```python
from build123d import *

# Parameters (mm, degrees)
F1_DEPTH = 0.5
F4_SCALE = 3


with BuildPart() as f1:
    # F0 (on Top) → F1 (new body)
    with BuildSketch(Plane.XY):
        with BuildLine():
            ThreePointArc((0.6081234737, 2.1142814502), (-0.4630317257, 1.4250651194), (-1.7347256805, 1.3530436147))
            ThreePointArc((-1.7347256805, 1.3530436147), (-1.7798374262, 1.2931275831), (-1.8228806624, 1.2317086913))
            ThreePointArc((-1.8228806624, 1.2317086913), (-1.4984021401, 0), (-1.8228806624, -1.2317086913))
            ThreePointArc((-1.8228806624, -1.2317086913), (-1.7798374262, -1.2931275831), (-1.7347256805, -1.3530436147))
            ThreePointArc((-1.7347256805, -1.3530436147), (-0.4646832841, -1.4263763437), (0.6048373994, -2.1152238487))
            ThreePointArc((0.6048373994, -2.1152238487), (0.6802746399, -2.0921822636), (0.7548374053, -2.0664512337))
            ThreePointArc((0.7548374053, -2.0664512337), (1.2149085882, -0.8808585803), (2.1987212669, -0.075000003))
            ThreePointArc((2.1987212669, -0.075000003), (2.2000000477, 0), (2.1987212669, 0.075000003))
            ThreePointArc((2.1987212669, 0.075000003), (1.2122351514, 0.8807449808), (0.7507612307, 2.0679356335))
            ThreePointArc((0.7507612307, 2.0679356335), (0.6798374024, 2.0923243812), (0.6081234737, 2.1142814502))
        make_face()
        with BuildLine():
            ThreePointArc((-1.0484390882, 0.5341534637), (1.1766666667, 0), (-1.0484390882, -0.5341534637))
            ThreePointArc((-1.0484390882, -0.5341534637), (-1.0581051368, -0.4731125583), (-1.0300472939, -0.4180473054))
            Line((-1.0300472939, -0.4180473054), (-0.7534213469, -0.1414213583))
            ThreePointArc((-0.7534213469, -0.1414213583), (-0.6948427023, 0), (-0.7534213469, 0.1414213583))
            Line((-0.7534213469, 0.1414213583), (-1.0300472939, 0.4180473054))
            ThreePointArc((-1.0300472939, 0.4180473054), (-1.0581051368, 0.4731125583), (-1.0484390882, 0.5341534637))
        make_face(mode=Mode.SUBTRACT)
    extrude(amount=F1_DEPTH)

    # F2 (on Front) → F3 (revolve, cut)
    with BuildSketch(Plane.XZ):
        Polygon((1.85, 0.5), (1.6, 0.5), (1.6, 0.3556624327), align=None)
    revolve(axis=Axis((1.6, 0, 0.4278312164), (0, 0, -1)), mode=Mode.SUBTRACT)


with BuildPart() as f1_1:
    # F4: moved
    add(f1.part.scale(F4_SCALE))


solid = f1_1.part
```
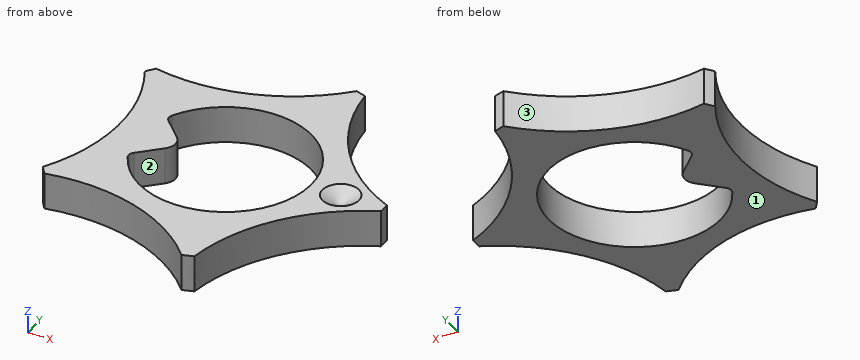
Part model, mm, in its own coordinate system. Face numbers are marked on the shaded views. Round coordinates to 2 decimals unless told otherwise and drop trailing zeros. Order: outer loops, then holes, each group sorted by start corner. A loop starts at its lowest first (then second) coordinate and runs counter-clockwise, first axis right, second up. Notation, with made-up numbers: M 6.5,77.25 L 33.5,77.25 A19 cw 33.5,81.25 Z; hole C 70.5,50 d10. An arc over 180 degrees is marked long. Put each result on its own line as item: value. Start each with the question number.
1. Drill centre lines: probe 1 along X at (y, z) = (0, 0.3); probe 2 along Y at (x, z) = (0.25, 1.1); probe 3 along Y at (x, z) = (0, 0.55). Where is each one in solid material? Low to high. Write a range as [from, to].
2. Slice it at D-D on z = 1.35. List the corners of the cut face in (x, y) (3 decimals).
3. Two-plate mould, pull along Y, no slides. Class the marked faces 1, 2 and 3: +Y half, -Y half, draft (parallel to the pull), parting line (faces both ways), or undercut.
4. Slice it at A-A on y = 2.25. List the corners of the cut face in (x, z), then the cut area to 3 significant figures.
5. Slice it at C-C on z = 0.5. List the corners of the cut face in (x, y) (3 decimals), then the cut area to 3 significant figures.
6. Slice it at B-B on x = 2.75. List the corners of the cut face in (y, z).
Findings:
1. probe 1: [-4.5, -2.08], [3.53, 6.6]
1. probe 2: [-5.05, -3.52], [3.52, 5.04]
1. probe 3: [-4.9, -3.53], [3.53, 4.89]
2. outline: M -5.469,-3.695 A6.6 ccw -5.204,-4.059 A7.5 cw 1.815,-6.346 A6.6 ccw 2.265,-6.199 A7.5 cw 6.596,-0.225 A6.6 ccw 6.596,0.225 A7.5 cw 2.252,6.204 A6.6 ccw 1.824,6.343 A7.5 cw -5.204,4.059 A6.6 ccw -5.469,3.695 A7.5 cw Z; hole M -3.145,-1.602 A3.53 ccw long -3.145,1.602 A0.3 ccw -3.09,1.254 L -2.26,0.424 A0.6 cw -2.26,-0.424 L -3.09,-1.254 A0.3 ccw Z; hole C 4.8,0 d0.98
3. face 1: draft
3. face 2: undercut
3. face 3: +Y half
4. outline: M -4.84,0 L -2.72,0 L -2.72,1.5 L -4.84,1.5 Z; M 2.72,0 L 3.94,0 L 3.94,1.5 L 2.72,1.5 Z
4. area: 5.01 mm2
5. outline: M -5.469,-3.695 A6.6 ccw -5.204,-4.059 A7.5 cw 1.815,-6.346 A6.6 ccw 2.265,-6.199 A7.5 cw 6.596,-0.225 A6.6 ccw 6.596,0.225 A7.5 cw 2.252,6.204 A6.6 ccw 1.824,6.343 A7.5 cw -5.204,4.059 A6.6 ccw -5.469,3.695 A7.5 cw Z; hole M -3.145,-1.602 A3.53 ccw long -3.145,1.602 A0.3 ccw -3.09,1.254 L -2.26,0.424 A0.6 cw -2.26,-0.424 L -3.09,-1.254 A0.3 ccw Z
5. area: 47.6 mm2
6. outline: M -4.27,0 L -2.21,0 L -2.21,1.5 L -4.27,1.5 Z; M 2.21,0 L 4.24,0 L 4.24,1.5 L 2.21,1.5 Z
